Verification items for the finished model (mm, model axes). Face numbers are marked on the shaded views. A direction names the side the tool comes from. Give positions to 0.01 mm unless a question says otherwise; leave off trailing zeros. Loops run counter-clockwise (first coordinate to the right, second up) from the corner with the lowest first, then second, coordinate; pieces in that order, holes last. Notation, with made-up numbers: (46.25, 1) - (100.25, 1) arc R27 ccw to (100.25, 30) - close; hole circle Ø11 at (-19, 43). An arc over 180 degrees is marked (long way). One line per item, written item: value. Start each with the question number.
1. Scan lines: L1, parallel to Z at x = -6, y = -15.5; L2, parallel to Z at x = -1, y = -37; L3, parallel to X at y = -21.35, z = 7.3. Record each from-to range of solid material in increasing order. Write a range as [from, to].
2. Mould release check, pull along X, two halves, no side actions. Record for the marked faces 1, 2 and 3: pulls with the +X half, pulls with the -X half, needs draft (parallel to the pull), parting line crosses it, or undercut.
3. Gauge pin test, flat ends, axial feed: pin 1 (5 mm diameter, centred on x = -8.5, z = -41.5, fed in from +Y); pin 2 (3.5 mm diameter, centred on x = 14.68, y = 1.14, fed in from +Z); pin 3 (3 mm diameter, centred on x = -1, z = 5, fed in from +Y); pin 4 (12 mm diameter, centred on y = -2.5, z = -7.5, fed in from -X). Record the tip position at first contact, or that the pin passes through.
4. Sectioned sample at A-A (y = -37). Record the cut outline in (x, z), plus the area to 3 significant figures.
5. Sectioned sample at C-C (y = 10.5). Record the cut outline in (x, z).
6. Sectioned sample at B-B (z = 1). Record the cut outline in (x, y), plus the area to 3 significant figures.
7. Access from +Z, -Z, +X, -X, +Y, -Y to the whole of each face (thin tool, end or side, straight path). Record for the marked faces 4, 5 and 6.
from build123d import *

# Parameters (mm, degrees)
SKETCH_1_W           = 38
SKETCH_1_H           = 45
SKETCH_1_R           = 1.6
EXTRUDE_1_DEPTH      = 2.5
CUT_EXTRUDE_1_DEPTH  = 2.5
SKETCH_3_W           = 38
SKETCH_3_H           = 55
EXTRUDE_2_DEPTH      = 2.5
FILLET_3_R           = 1
FILLET1_R            = 5
EXTRUDE3_DEPTH       = 2
LPATTERN1_COUNT      = 4
LPATTERN1_PITCH      = 10
MIRROR3_COPY_1_DEPTH = 2
MIRROR3_COPY_2_DEPTH = 2
MIRROR3_COPY_3_DEPTH = 2
EXTRUDE4_DEPTH       = 5
EXTRUDE4_DEPTH_BACK  = 5
SKETCH5_W            = 8
SKETCH5_H            = 4
SKETCH6_R            = 1.6
CUT_EXTRUDE1_DEPTH   = 20
FILLET2_R            = 5
FILLET3_R            = 5


with BuildPart() as part:
    # 草图1 → 凸台-拉伸1 (new body)
    with BuildSketch(Plane.XY):
        with Locations((-0.320113314, 1.635589826)):
            Rectangle(SKETCH_1_W, SKETCH_1_H)
        with Locations((-15.320113314, 21.135589826)):
            Circle(SKETCH_1_R, mode=Mode.SUBTRACT)
        with Locations((14.679886686, 21.135589826)):
            Circle(SKETCH_1_R, mode=Mode.SUBTRACT)
        with Locations((-15.320113314, 1.135589826)):
            Circle(SKETCH_1_R, mode=Mode.SUBTRACT)
        with Locations((14.679886686, 1.135589826)):
            Circle(SKETCH_1_R, mode=Mode.SUBTRACT)
    extrude_1 = extrude(amount=EXTRUDE_1_DEPTH)

    # 草图2 → 切除-拉伸1 (cut)
    with BuildSketch(Plane.XY.offset(2.5)):
        Polygon((-11.820113314, 24.135589826), (11.179886686, 24.135589826), (13.179886686, 24.135589826), (11.179886686, 22.135589826), (11.179886686, 12.135589826), (-11.820113314, 12.135589826), (-11.820113314, 22.135589826), (-13.820113314, 24.135589826), align=None)
    cut_extrude_1 = extrude(amount=-CUT_EXTRUDE_1_DEPTH, mode=Mode.SUBTRACT)

    # 草图3 → 凸台-拉伸2 (add)
    with BuildSketch(Plane.XZ.offset(20.864410174)):
        with Locations((-0.320113314, -25)):
            Rectangle(SKETCH_3_W, SKETCH_3_H)
    extrude(amount=EXTRUDE_2_DEPTH)

    # 圆角3
    fillet_3_edges = [part.edges().sort_by_distance(p)[0] for p in [
        (-13.820113314, 24.135589826, 1.25),
        (13.179886686, 24.135589826, 1.25),
        (11.179886686, 22.135589826, 1.25),
        (-11.820113314, 22.135589826, 1.25),
        (-19.320113314, 24.135589826, 1.25),
        (18.679886686, 24.135589826, 1.25),
    ]]
    fillet(fillet_3_edges, radius=FILLET_3_R)

    # Fillet1
    fillet1_edges = [part.edges().sort_by_distance(p)[0] for p in [
        (11.179886686, 12.135589826, 1.25),
        (-11.820113314, 12.135589826, 1.25),
    ]]
    fillet(fillet1_edges, radius=FILLET1_R)

    # Sketch4 → Extrude3 (add)
    with BuildSketch(Plane.ZY.offset(19.320113314)):
        with BuildLine():
            Line((0, -5.864410174), (0, -20.864410174))
            Line((0, -20.864410174), (-15, -20.864410174))
            ThreePointArc((-15, -20.864410174), (-4.393398282, -16.471011892), (0, -5.864410174))
        make_face()
    extrude3 = extrude(amount=-EXTRUDE3_DEPTH)

    # Mirror1: 凸台-拉伸1 across plane
    add(extrude_1.mirror(Plane(origin=(0, 0, -25), x_dir=(1, 0, 0), z_dir=(0, 0, -1))))

    # Mirror2: 切除-拉伸1 across plane
    add(cut_extrude_1.mirror(Plane(origin=(0, 0, -25), x_dir=(1, 0, 0), z_dir=(0, 0, -1))), mode=Mode.SUBTRACT)

    # LPattern1: Extrude3 ×4
    with Locations(*[(i * LPATTERN1_PITCH, 0, 0) for i in range(1, LPATTERN1_COUNT)]):
        add(extrude3)

    # Mirror3: Extrude3 across plane
    add(extrude3.mirror(Plane(origin=(0, 0, -25), x_dir=(1, 0, 0), z_dir=(0, 0, -1))))

    # Mirror3 copy 1 sketch → Mirror3 copy 1 (add)
    with BuildSketch(Plane(origin=(-9.320113314, 0, -50), x_dir=(0, 0, -1), z_dir=(-1, 0, 0))):
        with BuildLine():
            Line((0, 5.864410174), (0, 20.864410174))
            Line((0, 20.864410174), (-15, 20.864410174))
            ThreePointArc((-15, 20.864410174), (-4.393398282, 16.471011892), (0, 5.864410174))
        make_face()
    extrude(amount=-MIRROR3_COPY_1_DEPTH)

    # Mirror3 copy 2 sketch → Mirror3 copy 2 (add)
    with BuildSketch(Plane(origin=(0.679886686, 0, -50), x_dir=(0, 0, -1), z_dir=(-1, 0, 0))):
        with BuildLine():
            Line((0, 5.864410174), (0, 20.864410174))
            Line((0, 20.864410174), (-15, 20.864410174))
            ThreePointArc((-15, 20.864410174), (-4.393398282, 16.471011892), (0, 5.864410174))
        make_face()
    extrude(amount=-MIRROR3_COPY_2_DEPTH)

    # Mirror3 copy 3 sketch → Mirror3 copy 3 (add)
    with BuildSketch(Plane(origin=(10.679886686, 0, -50), x_dir=(0, 0, -1), z_dir=(-1, 0, 0))):
        with BuildLine():
            Line((0, 5.864410174), (0, 20.864410174))
            Line((0, 20.864410174), (-15, 20.864410174))
            ThreePointArc((-15, 20.864410174), (-4.393398282, 16.471011892), (0, 5.864410174))
        make_face()
    extrude(amount=-MIRROR3_COPY_3_DEPTH)

    # Sketch5 → Extrude4 (add, two sides: drawn at the far end of the back side and taken through both)
    with BuildSketch(Plane.ZY.offset(0.320113314).offset(-EXTRUDE4_DEPTH_BACK)):
        Polygon((-48.5, -23.364410174), (-48.5, -45.648790241), (-39.095261683, -54.441591814), (-32.049269501, -57.2068117), (-17.950730499, -57.2068117), (-10.904738317, -54.441591814), (-1.5, -45.648790241), (-1.5, -24.364410174), (10.5, -24.364410174), (10.5, -28.364410174), (2.5, -28.364410174), (2.5, -47.384968523), (-8.731572968, -57.885738362), (-17.193922344, -61.2068117), (-32.806077656, -61.2068117), (-41.268427032, -57.885738362), (-52.5, -47.384968523), (-52.5, -23.364410174), align=None)
        with Locations((6.5, -21.364410174)):
            Rectangle(SKETCH5_W, SKETCH5_H)
    extrude(amount=EXTRUDE4_DEPTH + EXTRUDE4_DEPTH_BACK)

    # Sketch6 → Cut-Extrude1 (cut)
    with BuildSketch(Plane.XZ.offset(28.364410174)):
        with Locations(Location((-0.320113314, 7.3, 0), (0, 0, 270))):
            Circle(SKETCH6_R)
    extrude(amount=-CUT_EXTRUDE1_DEPTH, mode=Mode.SUBTRACT)

    # Fillet2
    fillet2_edges = [part.edges().sort_by_distance(p)[0] for p in [
        (4.679886686, -23.364410174, -50.5),
        (-5.320113314, -23.364410174, -50.5),
    ]]
    fillet(fillet2_edges, radius=FILLET2_R)

    # Fillet3
    fillet3_edges = [part.edges().sort_by_distance(p)[0] for p in [
        (4.679886686, -21.364410174, 2.5),
        (-5.320113314, -21.364410174, 2.5),
    ]]
    fillet(fillet3_edges, radius=FILLET3_R)


solid = part.part
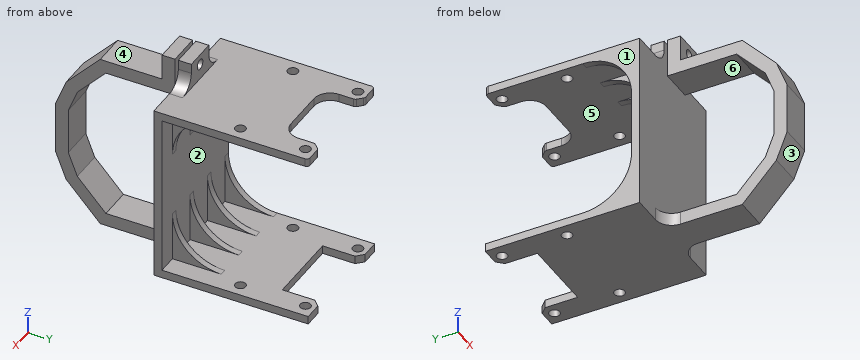
Results are:
1. L1: z = [-52.5, -50], [0, 2.5]
1. L2: z = [-52.5, -48.5], [-1.5, 2.5]
1. L3: x = [-5.32, -1.92], [1.28, 4.68]
2. face 1: pulls with the -X half
2. face 2: undercut
2. face 3: needs draft
3. pin 1: stops at y = -17.86
3. pin 2: stops at z = 2.5
3. pin 3: stops at y = -19.36
3. pin 4: passes through
4. outline: (-5.32, -52.5) - (4.68, -52.5) - (4.68, -48.5) - (-5.32, -48.5) - close; (-5.32, -1.5) - (4.68, -1.5) - (4.68, 2.5) - (-5.32, 2.5) - close
4. area: 80.0 mm^2
5. outline: (-19.32, -52.5) - (18.68, -52.5) - (18.68, -50) - (-19.32, -50) - close; (-19.32, 0) - (18.68, 0) - (18.68, 2.5) - (-19.32, 2.5) - close
6. outline: (-19.32, -23.36) - (18.68, -23.36) - (18.68, 23.14) arc R1 ccw to (17.68, 24.14) - (13.59, 24.14) arc R1 ccw to (12.89, 23.84) - (11.47, 22.43) arc R1 ccw to (11.18, 21.72) - (11.18, 17.14) arc R5 cw to (6.18, 12.14) - (-6.82, 12.14) arc R5 cw to (-11.82, 17.14) - (-11.82, 21.72) arc R1 ccw to (-12.11, 22.43) - (-13.53, 23.84) arc R1 ccw to (-14.23, 24.14) - (-18.32, 24.14) arc R1 ccw to (-19.32, 23.14) - close; (-5.32, -48.79) - (4.68, -48.79) - (4.68, -24.36) - (-5.32, -24.36) - close; hole circle Ø3.2 at (-15.32, 1.14); hole circle Ø3.2 at (-15.32, 21.14); hole circle Ø3.2 at (14.68, 1.14); hole circle Ø3.2 at (14.68, 21.14)
6. area: 1,750 mm^2
7. face 4: +Z, +X, -X, -Y
7. face 5: +Y
7. face 6: +X, -X
